Geometry: final body of the model. Coordinates: model frame, mm. A direction names the side the tool comes from. Round coordinates to 2 decimals unless told otherwise and drop trailing zeros. Order: outer loops, then holes, each group sorted by start corner. A loop starts at its lowest first (then second) coordinate and runs counter-clockwise, first axis right, second up. Notation, with made-up numbers: M 32.5,-21.75 L 44.5,-21.75 A20 cw 44.5,-10.75 Z; hole C 43,30.5 d10. An arc over 180 degrees is marked long. Return JSON: item names as keys, results as strings. Group by question number.
Q1. Cut plane A-A on x = 0. Output: boundary loops of the cut face in (y, z).
Q2. Contact query for a flat-ended pin moving along its axis: pin 1 (8 mm diameter, centred on x = 31.9, z = -0.7, fed in from +Y). Output: stop coordinate, or through.
Q3. Cut plane C-C on y = -1.5. Count the separate pieces of the cut face and the enclosed holes in it, and give its area (3 significant figures).
Q4. Cut plane B-B on z = -101. Output: boundary loops of the cut face in (x, y).
Q5. Mould query, pull axis X, two halves, no side actions, for faces 4 (the face through (-0.275, -2.465, 132.137)), 5 (the face through (19, -10, 2)), 6 (the face through (45, -5, -2)). Classes: released by +X, released by -X, zero draft, split by the parting line, or undercut.
Q6. Ray query, probe 1 along Z at (x, y) = (-31, -0.5); probe 2 along Z at (x, y) = (-1, -6.5); probe 3 along X at (y, z) = (-4, 104). Return the intervals inside material, ascending.
Q7. Access query for faces 1 (the face through (-45, -5, -2)), 2 (the face through (-13, -5, 1)), 3 (the face through (-12.5, -2, -2)). Directions: +Z, -Z, +X, -X, +Y, -Y. A direction counts if a zero-diameter tool reaches every point of the face in a straight line with its end or side. Return the directions, or none.
Q8. Cut plane D-D on x = -30.5. Output: boundary loops of the cut face in (y, z).
```python
from build123d import *

# Parameters (mm, degrees)
F0_W     = 90
F0_H     = 314.28
F1_DEPTH = 10
F3_DEPTH = 5
F4_R     = 4.5
F5_DEPTH = 25


with BuildPart() as f1:
    # F0 (on Front) → F1 (new body)
    with BuildSketch(Plane.XZ):
        Rectangle(F0_W, F0_H)
        with BuildLine():
            Line((-12.5, -119.64), (-12.5, 119.64))
            ThreePointArc((-12.5, 119.64), (0, 132.14), (12.5, 119.64))
            Line((12.5, 119.64), (12.5, -119.64))
            ThreePointArc((12.5, -119.64), (0, -132.14), (-12.5, -119.64))
        make_face(mode=Mode.SUBTRACT)
    extrude(amount=F1_DEPTH)

    # F2 (on face) → F3 (cut)
    with BuildSketch(Plane.XZ.offset(10)):
        with BuildLine():
            Line((17.5, -119.64), (17.5, 119.64))
            ThreePointArc((17.5, 119.64), (0, 137.14), (-17.5, 119.64))
            Line((-17.5, 119.64), (-17.5, -119.64))
            ThreePointArc((-17.5, -119.64), (0, -137.14), (17.5, -119.64))
        make_face()
    extrude(amount=-F3_DEPTH, mode=Mode.SUBTRACT)

    # F4 (on face) → F5 (cut)
    with BuildSketch(Plane.XZ.offset(10)):
        with Locations((31.899736, -112.695811)):
            Circle(F4_R)
        with Locations((-30.900264, -112.695811)):
            Circle(F4_R)
        with Locations((31.899736, -56.695811)):
            Circle(F4_R)
        with Locations((31.899736, -0.695811)):
            Circle(F4_R)
        with Locations((31.899736, 55.304189)):
            Circle(F4_R)
        with Locations((31.899736, 111.304189)):
            Circle(F4_R)
        with Locations((-30.900264, 111.304189)):
            Circle(F4_R)
        with Locations((-30.900264, 55.304189)):
            Circle(F4_R)
        with Locations((-30.900264, -0.695811)):
            Circle(F4_R)
        with Locations((-30.900264, -56.695811)):
            Circle(F4_R)
    extrude(amount=-F5_DEPTH, mode=Mode.SUBTRACT)


solid = f1.part
```
Result sheet:
{
 "1": {"outline": "M -10,-157.14 L 0,-157.14 L 0,-132.14 L -5,-132.14 L -5,-137.14 L -10,-137.14 Z; M -10,137.14 L -5,137.14 L -5,132.14 L 0,132.14 L 0,157.14 L -10,157.14 Z"},
 "2": {"pin 1": "passes through"},
 "3": {"separate pieces": "1", "enclosed holes": "11", "area": "21,200 mm²"},
 "4": {"outline": "M -45,-10 L -17.5,-10 L -17.5,-5 L -12.5,-5 L -12.5,0 L -45,0 Z; M 12.5,-5 L 17.5,-5 L 17.5,-10 L 45,-10 L 45,0 L 12.5,0 Z"},
 "5": {"face 4": "undercut", "face 5": "zero draft", "face 6": "released by +X"},
 "6": {"probe 1": "z = -157.14 to -117.19, -108.2 to -61.19, -52.2 to -5.19, 3.8 to 50.81, 59.8 to 106.81, 115.8 to 157.14", "probe 2": "z = -157.14 to -137.11, 137.11 to 157.14", "probe 3": "x = -45 to -12.5, 12.5 to 45"},
 "7": {"face 1": "+Z, -Z, -X, +Y, -Y", "face 2": "-Y", "face 3": "+Y, -Y"},
 "8": {"outline": "M -10,-157.14 L 0,-157.14 L 0,-117.18 L -10,-117.18 Z; M -10,-108.21 L 0,-108.21 L 0,-61.18 L -10,-61.18 Z; M -10,-52.21 L 0,-52.21 L 0,-5.18 L -10,-5.18 Z; M -10,3.79 L 0,3.79 L 0,50.82 L -10,50.82 Z; M -10,59.79 L 0,59.79 L 0,106.82 L -10,106.82 Z; M -10,115.79 L 0,115.79 L 0,157.14 L -10,157.14 Z"}
}
